Part model, mm, in its own coordinate system. Face numbers are marked on the shaded views. Give positions to 0.01 mm unless a question says otherwise; leave off trailing zeros. Write each loop counter-clockwise with the first axis right and the second up, starting at its lowest first coordinate (ties: lowest second). Pieces come first, ordered by that corner, then holes.
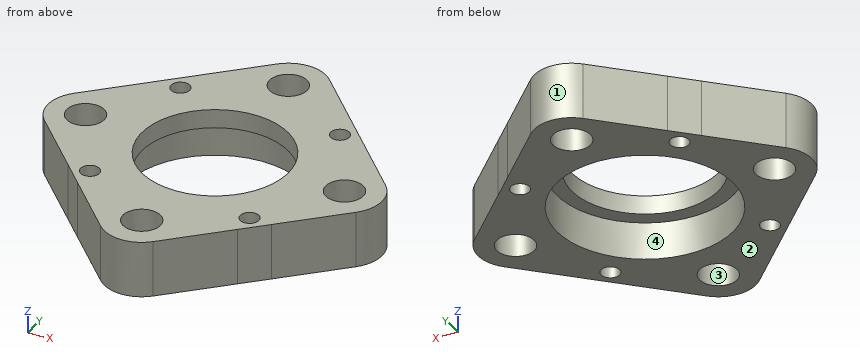
from build123d import *

# Parameters (mm, degrees)
SZKIC1_R                    = 35
SZKIC1_R_2                  = 23.5
SZKIC1_R_3                  = 19.5
DODANIE_WYCI_GNI_CIE3_DEPTH = 5
DODANIE_WYCI_GNI_CIE5_START = 10
SZKIC4_R                    = 35
SZKIC4_R_2                  = 23.5
DODANIE_WYCI_GNI_CIE5_DEPTH = 10
SZKIC13_R                   = 10
DODANIE_WYCI_GNI_CIE6_DEPTH = 15
OTWORY_USTALAJ_CE_10_0MM1_D = 10
OTWORY_USTALAJ_CE_5_0MM3_D  = 5
DODANIE_WYCI_GNI_CIE7_DEPTH = 15
SZKIC28_R                   = 52.509364788
WYTNIJ_WYCI_GNI_CIE6_DEPTH  = 15


with BuildPart() as part:
    # Szkic1 → Dodanie-wyciągnięcie3 (new body)
    # profile 1 of 2: a face of its own
    with BuildSketch(Plane.XY):
        Circle(SZKIC1_R)
        Circle(SZKIC1_R_2, mode=Mode.SUBTRACT)
    # profile 2 of 2: a face of its own
    with BuildSketch(Plane.XY):
        Circle(SZKIC1_R_2)
        Circle(SZKIC1_R_3, mode=Mode.SUBTRACT)
    extrude(amount=DODANIE_WYCI_GNI_CIE3_DEPTH)

    # Szkic4 → Dodanie-wyciągnięcie5 (add)
    with BuildSketch(Plane(origin=(0, 0, 0), x_dir=(-1, 0, 0), z_dir=(0, 0, -1)).offset(DODANIE_WYCI_GNI_CIE5_START)):
        Circle(SZKIC4_R)
        Circle(SZKIC4_R_2, mode=Mode.SUBTRACT)
    extrude(amount=-DODANIE_WYCI_GNI_CIE5_DEPTH)

    # Szkic13 → Dodanie-wyciągnięcie6 (add)
    with BuildSketch(Plane(origin=(0, 0, -10), x_dir=(-1, 0, 0), z_dir=(0, 0, -1))):
        with Locations((0, 35)):
            Circle(SZKIC13_R)
        with Locations((0, -35)):
            Circle(SZKIC13_R)
        with Locations((-35, 0)):
            Circle(SZKIC13_R)
        with Locations((35, 0)):
            Circle(SZKIC13_R)
    extrude(amount=-DODANIE_WYCI_GNI_CIE6_DEPTH)

    # Otwory ustalające Ø10.0mm1 (through all)
    with Locations(Plane.XY.offset(5)):
        with Locations((0, 35), (0, -35), (-35, 0), (35, 0)):
            Hole(OTWORY_USTALAJ_CE_10_0MM1_D / 2)

    # Otwory ustalające Ø5.0mm3 (through all)
    with Locations(Plane.XY.offset(5)):
        with Locations((-21.566756826, 21.566756826), (21.566756826, 21.566756826), (21.566756826, -21.566756826), (-21.566756826, -21.566756826)):
            Hole(OTWORY_USTALAJ_CE_5_0MM3_D / 2)

    # Szkic27 → Dodanie-wyciągnięcie7 (add)
    with BuildSketch(Plane(origin=(0, 0, -10), x_dir=(-1, 0, 0), z_dir=(0, 0, -1))):
        with BuildLine():
            ThreePointArc((33.571428571, 9.897433186), (38.155396436, 9.48912395), (42.071067812, 7.071067812))
            Line((42.071067812, 7.071067812), (27.531241216, 21.610894407))
            ThreePointArc((27.531241216, 21.610894407), (31.107641461, 16.041029978), (33.571428571, 9.897433186))
        make_face()
        with BuildLine():
            ThreePointArc((9.897433186, 33.571428571), (16.041029978, 31.107641461), (21.610894407, 27.531241216))
            Line((21.610894407, 27.531241216), (7.071067812, 42.071067812))
            ThreePointArc((7.071067812, 42.071067812), (9.48912395, 38.155396436), (9.897433186, 33.571428571))
        make_face()
        with BuildLine():
            ThreePointArc((-9.897433186, 33.571428571), (-9.48912395, 38.155396436), (-7.071067812, 42.071067812))
            Line((-7.071067812, 42.071067812), (-21.610894407, 27.531241216))
            ThreePointArc((-21.610894407, 27.531241216), (-16.041029978, 31.107641461), (-9.897433186, 33.571428571))
        make_face()
        with BuildLine():
            ThreePointArc((-33.571428571, 9.897433186), (-31.107641461, 16.041029978), (-27.531241216, 21.610894407))
            Line((-27.531241216, 21.610894407), (-42.071067812, 7.071067812))
            ThreePointArc((-42.071067812, 7.071067812), (-38.155396436, 9.48912395), (-33.571428571, 9.897433186))
        make_face()
        with BuildLine():
            Line((-42.071067812, -7.071067812), (-27.531241216, -21.610894407))
            ThreePointArc((-27.531241216, -21.610894407), (-31.107641461, -16.041029978), (-33.571428571, -9.897433186))
            ThreePointArc((-33.571428571, -9.897433186), (-38.155396436, -9.48912395), (-42.071067812, -7.071067812))
        make_face()
        with BuildLine():
            Line((-21.610894407, -27.531241216), (-7.071067812, -42.071067812))
            ThreePointArc((-7.071067812, -42.071067812), (-9.48912395, -38.155396436), (-9.897433186, -33.571428571))
            ThreePointArc((-9.897433186, -33.571428571), (-16.041029978, -31.107641461), (-21.610894407, -27.531241216))
        make_face()
        with BuildLine():
            Line((7.071067812, -42.071067812), (21.610894407, -27.531241216))
            ThreePointArc((21.610894407, -27.531241216), (16.041029978, -31.107641461), (9.897433186, -33.571428571))
            ThreePointArc((9.897433186, -33.571428571), (9.48912395, -38.155396436), (7.071067812, -42.071067812))
        make_face()
        with BuildLine():
            Line((27.531241216, -21.610894407), (42.071067812, -7.071067812))
            ThreePointArc((42.071067812, -7.071067812), (38.155396436, -9.48912395), (33.571428571, -9.897433186))
            ThreePointArc((33.571428571, -9.897433186), (31.107641461, -16.041029978), (27.531241216, -21.610894407))
        make_face()
    extrude(amount=-DODANIE_WYCI_GNI_CIE7_DEPTH)

    # Szkic28 → Wytnij-wyciągnięcie6 (cut)
    # profile 1 of 5: a face of its own
    with BuildSketch(Plane(origin=(0, 0, -10), x_dir=(-1, 0, 0), z_dir=(0, 0, -1))):
        Circle(SZKIC28_R)
        with BuildLine():
            Line((49.142135624, 0), (42.071067812, -7.071067812))
            Line((42.071067812, -7.071067812), (41.070360041, -8.071775583))
            Line((41.070360041, -8.071775583), (27.531241216, -21.610894407))
            ThreePointArc((27.531241216, -21.610894407), (24.748737342, -24.748737342), (21.610894407, -27.531241216))
            Line((21.610894407, -27.531241216), (7.071067812, -42.071067812))
            Line((7.071067812, -42.071067812), (0, -49.142135624))
            Line((0, -49.142135624), (-7.071067812, -42.071067812))
            Line((-7.071067812, -42.071067812), (-21.610894407, -27.531241216))
            ThreePointArc((-21.610894407, -27.531241216), (-24.748737342, -24.748737342), (-27.531241216, -21.610894407))
            Line((-27.531241216, -21.610894407), (-42.071067812, -7.071067812))
            Line((-42.071067812, -7.071067812), (-49.142135624, 0))
            Line((-49.142135624, 0), (-42.071067812, 7.071067812))
            Line((-42.071067812, 7.071067812), (-27.531241216, 21.610894407))
            ThreePointArc((-27.531241216, 21.610894407), (-24.748737342, 24.748737342), (-21.610894407, 27.531241216))
            Line((-21.610894407, 27.531241216), (-7.071067812, 42.071067812))
            Line((-7.071067812, 42.071067812), (0, 49.142135624))
            Line((0, 49.142135624), (7.071067812, 42.071067812))
            Line((7.071067812, 42.071067812), (21.610894407, 27.531241216))
            ThreePointArc((21.610894407, 27.531241216), (24.748737342, 24.748737342), (27.531241216, 21.610894407))
            Line((27.531241216, 21.610894407), (42.071067812, 7.071067812))
            Line((42.071067812, 7.071067812), (49.142135624, 0))
        make_face(mode=Mode.SUBTRACT)
    # profile 2 of 5: a face of its own
    with BuildSketch(Plane(origin=(0, 0, -10), x_dir=(-1, 0, 0), z_dir=(0, 0, -1))):
        with BuildLine():
            ThreePointArc((21.610894407, -27.531241216), (24.748737342, -24.748737342), (27.531241216, -21.610894407))
            Line((27.531241216, -21.610894407), (21.610894407, -27.531241216))
        make_face()
    # profile 3 of 5: a face of its own
    with BuildSketch(Plane(origin=(0, 0, -10), x_dir=(-1, 0, 0), z_dir=(0, 0, -1))):
        with BuildLine():
            ThreePointArc((-27.531241216, -21.610894407), (-24.748737342, -24.748737342), (-21.610894407, -27.531241216))
            Line((-21.610894407, -27.531241216), (-27.531241216, -21.610894407))
        make_face()
    # profile 4 of 5: a face of its own
    with BuildSketch(Plane(origin=(0, 0, -10), x_dir=(-1, 0, 0), z_dir=(0, 0, -1))):
        with BuildLine():
            Line((-27.531241216, 21.610894407), (-21.610894407, 27.531241216))
            ThreePointArc((-21.610894407, 27.531241216), (-24.748737342, 24.748737342), (-27.531241216, 21.610894407))
        make_face()
    # profile 5 of 5: a face of its own
    with BuildSketch(Plane(origin=(0, 0, -10), x_dir=(-1, 0, 0), z_dir=(0, 0, -1))):
        with BuildLine():
            Line((21.610894407, 27.531241216), (27.531241216, 21.610894407))
            ThreePointArc((27.531241216, 21.610894407), (24.748737342, 24.748737342), (21.610894407, 27.531241216))
        make_face()
    extrude(amount=-WYTNIJ_WYCI_GNI_CIE6_DEPTH, mode=Mode.SUBTRACT)


solid = part.part
1) Mould opens along Y. For the marked faces 1, 2, 3 and 4 say: +Y half, -Y half, draft (parallel to the pull), parting line (faces both ways), or undercut.
Check result:
face 1: +Y half
face 2: draft
face 3: undercut
face 4: undercut
2) Saw through at C-C (y = 12). Write the cut outline in (x, z).
Check result:
outline: (-37.14, -10) - (-20.21, -10) - (-20.21, 0) - (-15.37, 0) - (-15.37, 5) - (-37.14, 5) - close; (15.37, 0) - (20.21, 0) - (20.21, -10) - (37.14, -10) - (37.14, 5) - (15.37, 5) - close
3) Saw through at D-D (z = -5.75). State how many separate pieces and enclosed holes the cut face has, and give its area (3 significant figures).
Check result:
separate pieces: 1
enclosed holes: 9
area: 2,620 mm2
4) Saw through at A-A (y = 0). Write the cut outline in (x, z), and give its area (3 significant figures).
Check result:
outline: (-45, -10) - (-40, -10) - (-40, 5) - (-45, 5) - close; (-30, -10) - (-23.5, -10) - (-23.5, 0) - (-19.5, 0) - (-19.5, 5) - (-30, 5) - close; (19.5, 0) - (23.5, 0) - (23.5, -10) - (30, -10) - (30, 5) - (19.5, 5) - close; (40, -10) - (45, -10) - (45, 5) - (40, 5) - close
area: 385 mm2
5) Drill centre lines: L1, parallel to Y at x = 0, z = -5; L2, parallel to X at y = 1, z = -0.5; L3, parallel to X at y = -22, z = 3.5. Where is each one in solid material? Low to high.
Check result:
L1: y = -45 to -40, -30 to -23.5, 23.5 to 30, 40 to 45
L2: x = -44.95 to -39.9, -30.1 to -23.48, 23.48 to 30.1, 39.9 to 44.95
L3: x = -27.14 to -24.03, -19.1 to 19.1, 24.03 to 27.14
6) Flat gauge pins, fed straight in: P1, Ø4.5, axis at x = 21.57, y = -21.57, coming from the -Z side; P2, Ø1, axis at x = -12, z = -2.5, coming from the -Y side; P3, Ø8, axis at x = -21.57, y = 21.57, coming from the -Z side; P4, Ø8, axis at x = -20.5, z = -4, coming from the -Y side. Where does each tip first touch, or does it go through?
Check result:
P1: passes through
P2: stops at y = -37.64
P3: stops at z = -10
P4: stops at y = -32.64
